Input: part model. Units: mm. Frame: model coordinates. A direction names the side the tool comes from. Round coordinates to 2 decimals unless told otherwise and drop trailing zeros. Write each loop counter-clockwise with the first axis right and the second up, starting at its lowest first coordinate (ties: lowest second). Pieces come first, ordered by that corner, then holes. Notation, with made-up numbers: (-10, -13) - (23, -13) arc R28 cw to (23, 20) - close; hole circle Ø6 at (29, 6.25). An arc over 180 degrees is marked (long way). Use one line per item in the form item = value.
```python
from build123d import *

# Parameters (mm, degrees)
MOUNTING_BASE_DEPTH                             = 4
CSK_FOR_M3_FLAT_HEAD_MACHINE_SCREW2_D           = 3.4
CSK_FOR_M3_FLAT_HEAD_MACHINE_SCREW2_DEPTH       = 4
CSK_FOR_M3_FLAT_HEAD_MACHINE_SCREW2_CSINK_D     = 6.3
CSK_FOR_M3_FLAT_HEAD_MACHINE_SCREW2_CSINK_ANGLE = 90
CSK_FOR_M3_FLAT_HEAD_MACHINE_SCREW2_TIP         = 1.021463052
CSK_FOR_M3_FLAT_HEAD_MACHINE_SCREW1_D           = 3.4
CSK_FOR_M3_FLAT_HEAD_MACHINE_SCREW1_CSINK_D     = 6.3
CSK_FOR_M3_FLAT_HEAD_MACHINE_SCREW1_CSINK_ANGLE = 90
SKETCH12_OUTSIDE_W                              = 165.288
SKETCH12_OUTSIDE_H                              = 165.288
SKETCH12_OUTSIDE_W_2                            = 115
SKETCH12_OUTSIDE_H_2                            = 115
CUT_EXTRUDE2_DEPTH                              = 20
SKETCH19_R                                      = 40
SKETCH19_R_2                                    = 19
CUT_EXTRUDE4_DEPTH                              = 1.25
CUT_EXTRUDE5_START                              = -4
SKETCH19_3_R                                    = 40
SKETCH19_3_R_2                                  = 19
CUT_EXTRUDE5_DEPTH                              = 1.25
FILLET1_R                                       = 1.5


with BuildPart() as part:
    # Sketch1 → Mounting base (new body)
    with BuildSketch(Plane(origin=(0, 0, 0), x_dir=(1, 0, 0), z_dir=(0, 1, 0))):
        Polygon((-63.639610307, 0), (0, -63.639610307), (63.639610307, 0), (0, 63.639610307), align=None)
    extrude(amount=MOUNTING_BASE_DEPTH)

    # CSK for M3 Flat Head Machine Screw2
    with Locations(Plane(origin=(0, 0, 0), x_dir=(-1, 0, 0), z_dir=(0, -1, 0))):
        with Locations((51, 0), (0, -51), (-51, 0), (0, 51)):
            CounterSinkHole(CSK_FOR_M3_FLAT_HEAD_MACHINE_SCREW2_D / 2, CSK_FOR_M3_FLAT_HEAD_MACHINE_SCREW2_CSINK_D / 2, depth=CSK_FOR_M3_FLAT_HEAD_MACHINE_SCREW2_DEPTH, counter_sink_angle=CSK_FOR_M3_FLAT_HEAD_MACHINE_SCREW2_CSINK_ANGLE)
            with Locations((0, 0, -(CSK_FOR_M3_FLAT_HEAD_MACHINE_SCREW2_DEPTH + CSK_FOR_M3_FLAT_HEAD_MACHINE_SCREW2_TIP / 2))):  # 118° drill point
                Cone(0, CSK_FOR_M3_FLAT_HEAD_MACHINE_SCREW2_D / 2, CSK_FOR_M3_FLAT_HEAD_MACHINE_SCREW2_TIP, mode=Mode.SUBTRACT)

    # CSK for M3 Flat Head Machine Screw1 (through all)
    with Locations(Plane(origin=(0, 4, -7.5), x_dir=(0, 0, 1), z_dir=(0, 1, 0))):
        with Locations((0, 0), (7.5, 7.5), (15, 0), (7.5, -7.5)):
            CounterSinkHole(CSK_FOR_M3_FLAT_HEAD_MACHINE_SCREW1_D / 2, CSK_FOR_M3_FLAT_HEAD_MACHINE_SCREW1_CSINK_D / 2, counter_sink_angle=CSK_FOR_M3_FLAT_HEAD_MACHINE_SCREW1_CSINK_ANGLE)

    # Sketch12 outside → Cut-Extrude2 (cut)
    with BuildSketch(Plane(origin=(0, 0, 0), x_dir=(1, 0, 0), z_dir=(0, 1, 0))):
        Rectangle(SKETCH12_OUTSIDE_W, SKETCH12_OUTSIDE_H)
        Rectangle(SKETCH12_OUTSIDE_W_2, SKETCH12_OUTSIDE_H_2, mode=Mode.SUBTRACT)
    extrude(amount=CUT_EXTRUDE2_DEPTH, mode=Mode.SUBTRACT)

    # Sketch19 → Cut-Extrude4 (cut)
    with BuildSketch(Plane(origin=(0, 4, 0), x_dir=(1, 0, 0), z_dir=(0, 1, 0))):
        with Locations(Location((0, 0, 0), (0, 0, 270))):
            Circle(SKETCH19_R)
        with Locations(Location((0, 0, 0), (0, 0, 270))):
            Circle(SKETCH19_R_2, mode=Mode.SUBTRACT)
    extrude(amount=-CUT_EXTRUDE4_DEPTH, mode=Mode.SUBTRACT)

    # Sketch19<3> → Cut-Extrude5 (cut)
    with BuildSketch(Plane(origin=(0, 4, 0), x_dir=(1, 0, 0), z_dir=(0, 1, 0)).offset(CUT_EXTRUDE5_START)):
        with Locations(Location((0, 0, 0), (0, 0, 270))):
            Circle(SKETCH19_3_R)
        with Locations(Location((0, 0, 0), (0, 0, 270))):
            Circle(SKETCH19_3_R_2, mode=Mode.SUBTRACT)
    extrude(amount=CUT_EXTRUDE5_DEPTH, mode=Mode.SUBTRACT)

    # Fillet1
    # the kernel refuses this fillet: 1.5 mm, written as the material it adds along each edge
    with BuildSketch(Plane(origin=(0, 2.75, 0), x_dir=(0, 0, 1), z_dir=(-1, 0, 0))) as fillet1_piece_1:
        with BuildLine():
            CenterArc((38.520980054, 1.5), FILLET1_R, 270, 80.405931773)
            Line((38.520980054, 0), (38.520980054, -0.03))
            Line((38.520980054, -0.03), (40, -0.03))
            Line((40, -0.03), (40.03, 0))
            ThreePointArc((40.03, 0), (40.03, 0.625), (40.029580399, 1.245))
            Line((40.029580399, 1.245), (40, 1.25))
        make_face()
    revolve(axis=Axis((0, 2.75, 0), (0, 1, 0)))
    with BuildSketch(Plane(origin=(0, 2.75, 0), x_dir=(0, 0, 1), z_dir=(-1, 0, 0))) as fillet1_piece_2:
        with BuildLine():
            CenterArc((20.479019946, 1.5), FILLET1_R, 189.594068227, 80.405931773)
            Line((19, 1.25), (18.970419601, 1.245))
            ThreePointArc((18.970419601, 1.245), (18.97, 0.625), (18.97, 0))
            Line((18.97, 0), (19, -0.03))
            Line((19, -0.03), (20.479019946, -0.03))
            Line((20.479019946, -0.03), (20.479019946, 0))
        make_face()
    revolve(axis=Axis((0, 2.75, 0), (0, 1, 0)))
    with BuildSketch(Plane(origin=(0, 1.25, 0), x_dir=(0, 0, 1), z_dir=(-1, 0, 0))) as fillet1_piece_3:
        with BuildLine():
            CenterArc((38.520980054, -1.5), FILLET1_R, 9.594068227, 80.405931773)
            Line((38.520980054, 0), (38.520980054, 0.03))
            Line((38.520980054, 0.03), (40, 0.03))
            Line((40, 0.03), (40.03, 0))
            ThreePointArc((40.03, 0), (40.03, -0.625), (40.029580399, -1.245))
            Line((40.029580399, -1.245), (40, -1.25))
        make_face()
    revolve(axis=Axis((0, 1.25, 0), (0, 1, 0)))
    with BuildSketch(Plane(origin=(0, 1.25, 0), x_dir=(0, 0, 1), z_dir=(-1, 0, 0))) as fillet1_piece_4:
        with BuildLine():
            CenterArc((20.479019946, -1.5), FILLET1_R, 90, 80.405931773)
            Line((19, -1.25), (18.970419601, -1.245))
            ThreePointArc((18.970419601, -1.245), (18.97, -0.625), (18.97, 0))
            Line((18.97, 0), (19, 0.03))
            Line((19, 0.03), (20.479019946, 0.03))
            Line((20.479019946, 0.03), (20.479019946, 0))
        make_face()
    revolve(axis=Axis((0, 1.25, 0), (0, 1, 0)))


solid = part.part
```
(1) Draft query along Z for faces 4 (the face through (-1.03, 1.26, -6.15)), 5 (the face through (31.46, 1.97, 32.18)), 6 (the face through (32.18, 1.97, -31.46)). Return one class per face: released by +Z, released by -Z, zero draft, split by the parting line, or undercut.
Derived:
face_4 = undercut
face_5 = released by +Z
face_6 = released by -Z
(2) First-contact query: pin 1 Ø1.5 at (x, y) = (-43, 2.5) entering from +Z; pin 2 Ø4.5 at (x, z) = (7.5, 0) entering from +Y; pin 3 Ø12 at (x, z) = (-19.5, -25.5) entering from +Y. Flat tips, straight axial feed; report the tip coordinate or a pass-through.
Derived:
pin_1 = 21.39
pin_2 = 3.1
pin_3 = 2.75
(3) Cut plane A-A on z = -51. Output: boundary loops of the cut face in (x, y), then the cut area to 3 significant figures.
Derived:
outline = (-12.64, 0) - (-3.15, 0) - (-1.7, 1.45) - (-1.7, 4) - (-12.64, 4) - close; (1.7, 1.45) - (3.15, 0) - (12.64, 0) - (12.64, 4) - (1.7, 4) - close
area = 85.4 mm^2
(4) Material intervals for L1, parallel to Z at x = 0, y = 2; L2, parallel to Z at x = -9.5, y = 3.5; L3, parallel to Z at x = 6, y = 2.9, sorted ascending.
Derived:
L1 = -57.5 to -52.7, -49.3 to -9.2, -5.8 to 5.8, 9.2 to 49.3, 52.7 to 57.5
L2 = -54.14 to -38.67, -16.66 to -1.74, 1.74 to 16.66, 38.67 to 54.14
L3 = -57.5 to -38.71, -18.9 to -1.4, 1.4 to 18.9, 38.71 to 57.5
(5) Access query for faces 1 (the face through (-17, 1.25, 17)), 2 (the face through (-17, 2.75, 17)), 3 (the face through (-0.37, 2.74, 52.66)). Directions: +Z, -Z, +X, -X, +Y, -Y. A direction counts if a zero-diameter tool reaches every point of the face in a straight line with its end or side. Return the directions, or none.
Derived:
face_1 = -Y
face_2 = +Y
face_3 = +Y, -Y
